For this review, take the finished solid that the model builds, in its own axes (mm). A direction names the side the tool comes from. Round coordinates to 2 decimals unless told otherwise and drop trailing zeros. Write each loop counter-clockwise with the first axis right and the second up, starting at its lowest first coordinate (ties: lowest second). Pieces come first, ordered by that corner, then holes. Notation, with made-up numbers: (65.5, -15.75) -> (119.5, -15.75) arc R26 ccw to (119.5, 1.25) -> close; hole circle Ø8 at (-28, 86). An arc over 180 degrees is marked (long way). Answer in a Markdown table with one row per item. Add a question column.
```python
from build123d import *
from OCP.BRepFilletAPI import BRepFilletAPI_MakeChamfer
from build123d.topology import SkipClean

# Parameters (mm, degrees)
SKETCH1_R                 = 12
SKETCH1_R_2               = 8
BOSS_EXTRUDE4_DEPTH       = 2
BOSS_EXTRUDE5_START       = 2
SKETCH1_9_R               = 12
SKETCH1_9_R_2             = 9
BOSS_EXTRUDE5_DEPTH       = 4
BOSS_EXTRUDE6_START       = 2
BOSS_EXTRUDE6_DEPTH       = 2
BOSS_EXTRUDE7_START       = 4
BOSS_EXTRUDE7_DEPTH       = 2
BOSS_EXTRUDE8_START       = 4
SKETCH1_12_W              = 60
SKETCH1_12_H              = 60
SKETCH1_12_R              = 12
BOSS_EXTRUDE8_DEPTH       = 2
BOSS_EXTRUDE9_DEPTH       = 6
CHAMFER1_SIZE             = 1
CHAMFER1_SIZE2            = 0.176326981
BOSS_EXTRUDE10_DEPTH      = 6
BOSS_EXTRUDE11_DEPTH      = 20
BOSS_EXTRUDE12_DEPTH      = 2
BOSS_EXTRUDE12_DEPTH_BACK = 2
SKETCH1_14_R              = 8
CUT_EXTRUDE1_DEPTH        = 46.343136195


with BuildPart() as part:
    # Sketch1 → Boss-Extrude4 (new body)
    with BuildSketch(Plane(origin=(0, 0, 0), x_dir=(1, 0, 0), z_dir=(0, 1, 0))):
        with Locations(Location((0, 0, 0), (0, 0, 270))):
            Circle(SKETCH1_R)
        with Locations(Location((0, 0, 0), (0, 0, 270))):
            Circle(SKETCH1_R_2, mode=Mode.SUBTRACT)
    extrude(amount=BOSS_EXTRUDE4_DEPTH)

    # Sketch1<9> → Boss-Extrude5 (add)
    with BuildSketch(Plane(origin=(0, 0, 0), x_dir=(1, 0, 0), z_dir=(0, 1, 0)).offset(BOSS_EXTRUDE5_START)):
        with Locations(Location((0, 0, 0), (0, 0, 270))):
            Circle(SKETCH1_9_R)
        with Locations(Location((0, 0, 0), (0, 0, 270))):
            Circle(SKETCH1_9_R_2, mode=Mode.SUBTRACT)
    extrude(amount=BOSS_EXTRUDE5_DEPTH)

    # Sketch1<10> → Boss-Extrude6 (add)
    with SkipClean():  # the faces are left unmerged after this step: merging them gives an invalid solid
        with BuildSketch(Plane(origin=(0, 0, 0), x_dir=(1, 0, 0), z_dir=(0, 1, 0)).offset(BOSS_EXTRUDE6_START)):
            with BuildLine():
                ThreePointArc((0, 8), (2.070552361, 7.72740661), (4, 6.92820323))
                Line((4, 6.92820323), (4.5, 7.794228634))
                ThreePointArc((4.5, 7.794228634), (2.329371406, 8.693332437), (0, 9))
                Line((0, 9), (0, 8))
            make_face()
            with BuildLine():
                ThreePointArc((-8, 0), (-7.72740661, 2.070552361), (-6.92820323, 4))
                Line((-6.92820323, 4), (-7.794228634, 4.5))
                ThreePointArc((-7.794228634, 4.5), (-8.693332437, 2.329371406), (-9, 0))
                Line((-9, 0), (-8, 0))
            make_face()
            with BuildLine():
                Line((0, -9), (0, -8))
                ThreePointArc((0, -8), (-2.070552361, -7.72740661), (-4, -6.92820323))
                Line((-4, -6.92820323), (-4.5, -7.794228634))
                ThreePointArc((-4.5, -7.794228634), (-2.329371406, -8.693332437), (0, -9))
            make_face()
            with BuildLine():
                Line((9, 0), (8, 0))
                ThreePointArc((8, 0), (7.72740661, -2.070552361), (6.92820323, -4))
                Line((6.92820323, -4), (7.794228634, -4.5))
                ThreePointArc((7.794228634, -4.5), (8.693332437, -2.329371406), (9, 0))
            make_face()
        extrude(amount=BOSS_EXTRUDE6_DEPTH)

    # Sketch1<11> → Boss-Extrude7 (add)
    with SkipClean():  # the faces are left unmerged after this step: merging them gives an invalid solid
        with BuildSketch(Plane(origin=(0, 0, 0), x_dir=(1, 0, 0), z_dir=(0, 1, 0)).offset(BOSS_EXTRUDE7_START)):
            with BuildLine():
                ThreePointArc((0, 8), (2.070552361, 7.72740661), (4, 6.92820323))
                Line((4, 6.92820323), (4.5, 7.794228634))
                ThreePointArc((4.5, 7.794228634), (2.329371406, 8.693332437), (0, 9))
                Line((0, 9), (0, 8))
            make_face()
            with BuildLine():
                ThreePointArc((4, 6.92820323), (5.656854249, 5.656854249), (6.92820323, 4))
                Line((6.92820323, 4), (7.794228634, 4.5))
                ThreePointArc((7.794228634, 4.5), (6.363961031, 6.363961031), (4.5, 7.794228634))
                Line((4.5, 7.794228634), (4, 6.92820323))
            make_face()
            with BuildLine():
                ThreePointArc((-8, 0), (-7.72740661, 2.070552361), (-6.92820323, 4))
                Line((-6.92820323, 4), (-7.794228634, 4.5))
                ThreePointArc((-7.794228634, 4.5), (-8.693332437, 2.329371406), (-9, 0))
                Line((-9, 0), (-8, 0))
            make_face()
            with BuildLine():
                ThreePointArc((-6.92820323, 4), (-5.656854249, 5.656854249), (-4, 6.92820323))
                Line((-4, 6.92820323), (-4.5, 7.794228634))
                ThreePointArc((-4.5, 7.794228634), (-6.363961031, 6.363961031), (-7.794228634, 4.5))
                Line((-7.794228634, 4.5), (-6.92820323, 4))
            make_face()
            with BuildLine():
                Line((-4.5, -7.794228634), (-4, -6.92820323))
                ThreePointArc((-4, -6.92820323), (-5.656854249, -5.656854249), (-6.92820323, -4))
                Line((-6.92820323, -4), (-7.794228634, -4.5))
                ThreePointArc((-7.794228634, -4.5), (-6.363961031, -6.363961031), (-4.5, -7.794228634))
            make_face()
            with BuildLine():
                Line((0, -9), (0, -8))
                ThreePointArc((0, -8), (-2.070552361, -7.72740661), (-4, -6.92820323))
                Line((-4, -6.92820323), (-4.5, -7.794228634))
                ThreePointArc((-4.5, -7.794228634), (-2.329371406, -8.693332437), (0, -9))
            make_face()
            with BuildLine():
                Line((9, 0), (8, 0))
                ThreePointArc((8, 0), (7.72740661, -2.070552361), (6.92820323, -4))
                Line((6.92820323, -4), (7.794228634, -4.5))
                ThreePointArc((7.794228634, -4.5), (8.693332437, -2.329371406), (9, 0))
            make_face()
            with BuildLine():
                Line((7.794228634, -4.5), (6.92820323, -4))
                ThreePointArc((6.92820323, -4), (5.656854249, -5.656854249), (4, -6.92820323))
                Line((4, -6.92820323), (4.5, -7.794228634))
                ThreePointArc((4.5, -7.794228634), (6.363961031, -6.363961031), (7.794228634, -4.5))
            make_face()
        extrude(amount=BOSS_EXTRUDE7_DEPTH)

    # Sketch1<12> → Boss-Extrude8 (add)
    with SkipClean():  # the faces are left unmerged after this step: merging them gives an invalid solid
        with BuildSketch(Plane(origin=(0, 0, 0), x_dir=(1, 0, 0), z_dir=(0, 1, 0)).offset(BOSS_EXTRUDE8_START)):
            Rectangle(SKETCH1_12_W, SKETCH1_12_H)
            with Locations(Location((0, 0, 0), (0, 0, 270))):
                Circle(SKETCH1_12_R, mode=Mode.SUBTRACT)
        extrude(amount=BOSS_EXTRUDE8_DEPTH)

    # Sketch3 → Boss-Extrude9 (add)
    with SkipClean():  # the faces are left unmerged after this step: merging them gives an invalid solid
        with BuildSketch(Plane.XZ.offset(-4)):
            Polygon((-30, -30), (30, -30), (30, -28), (-28, -28), (-28, 30), (-30, 30), align=None)
            Polygon((30, -20), (30, -18), (-18, -18), (-18, 30), (-20, 30), (-20, -20), align=None)
        extrude(amount=BOSS_EXTRUDE9_DEPTH)

    # Chamfer1: one chamfer whose edges measure the first distance from different faces: ONE call of the kernel's chamfer builder (chamfer() names one face for all edges)
    chamfer1_edges_1 = [part.edges().sort_by_distance(p)[0] for p in [
        (-28, -2, 1),
    ]]
    chamfer1_side_1 = [part.faces().sort_by_distance(p)[0] for p in [
        (-28, 1, 1),
    ]]
    chamfer1_edges_2 = [part.edges().sort_by_distance(p)[0] for p in [
        (1, -2, -28),
    ]]
    chamfer1_side_2 = [part.faces().sort_by_distance(p)[0] for p in [
        (1, 1, -28),
    ]]
    chamfer1_edges_3 = [part.edges().sort_by_distance(p)[0] for p in [
        (-29, -2, 30),
    ]]
    chamfer1_side_3 = [part.faces().sort_by_distance(p)[0] for p in [
        (-29, 1, 30),
    ]]
    chamfer1_edges_4 = [part.edges().sort_by_distance(p)[0] for p in [
        (-30, -2, 0),
    ]]
    chamfer1_side_4 = [part.faces().sort_by_distance(p)[0] for p in [
        (-30, 1, 0),
    ]]
    chamfer1_edges_5 = [part.edges().sort_by_distance(p)[0] for p in [
        (0, -2, -30),
    ]]
    chamfer1_side_5 = [part.faces().sort_by_distance(p)[0] for p in [
        (0, 1, -30),
    ]]
    chamfer1_edges_6 = [part.edges().sort_by_distance(p)[0] for p in [
        (30, -2, -29),
    ]]
    chamfer1_side_6 = [part.faces().sort_by_distance(p)[0] for p in [
        (30, 1, -29),
    ]]
    chamfer1 = BRepFilletAPI_MakeChamfer(part.part.solid().wrapped)
    for e in chamfer1_edges_1:
        chamfer1.Add(CHAMFER1_SIZE, CHAMFER1_SIZE2, e.wrapped, chamfer1_side_1[0].wrapped)  # the first distance lies on this face
    for e in chamfer1_edges_2:
        chamfer1.Add(CHAMFER1_SIZE, CHAMFER1_SIZE2, e.wrapped, chamfer1_side_2[0].wrapped)  # the first distance lies on this face
    for e in chamfer1_edges_3:
        chamfer1.Add(CHAMFER1_SIZE, CHAMFER1_SIZE2, e.wrapped, chamfer1_side_3[0].wrapped)  # the first distance lies on this face
    for e in chamfer1_edges_4:
        chamfer1.Add(CHAMFER1_SIZE, CHAMFER1_SIZE2, e.wrapped, chamfer1_side_4[0].wrapped)  # the first distance lies on this face
    for e in chamfer1_edges_5:
        chamfer1.Add(CHAMFER1_SIZE, CHAMFER1_SIZE2, e.wrapped, chamfer1_side_5[0].wrapped)  # the first distance lies on this face
    for e in chamfer1_edges_6:
        chamfer1.Add(CHAMFER1_SIZE, CHAMFER1_SIZE2, e.wrapped, chamfer1_side_6[0].wrapped)  # the first distance lies on this face
    add(Compound.cast(chamfer1.Shape()), mode=Mode.REPLACE)

    # Sketch6 → Boss-Extrude10 (add)
    with BuildSketch(Plane.XZ.offset(-4)):
        Polygon((-18, 30), (-18, 28), (28, 28), (28, -18), (30, -18), (30, 30), align=None)
    extrude(amount=BOSS_EXTRUDE10_DEPTH)

    # Sketch3<3> → Boss-Extrude11 (add)
    with BuildSketch(Plane.XZ.offset(-4)):
        Polygon((-20, 30), (-20, -20), (-18, -18), (-18, 28), (-18, 30), align=None)
        Polygon((-20, -20), (30, -20), (30, -18), (28, -18), (-18, -18), align=None)
    extrude(amount=BOSS_EXTRUDE11_DEPTH)

    # Sketch9 → Boss-Extrude12 (add, two sides: drawn at the far end of the back side and taken through both)
    with BuildSketch(Plane(origin=(0, 0, 0), x_dir=(-0.7071067811865476, 0, -0.7071067811865475), z_dir=(0.7071067811865475, 0, -0.7071067811865476)).offset(-BOSS_EXTRUDE12_DEPTH_BACK)):
        Polygon((25.455844123, -16), (25.455844123, 0), (0, 0), align=None)
    extrude(amount=BOSS_EXTRUDE12_DEPTH + BOSS_EXTRUDE12_DEPTH_BACK)

    # Sketch1<14> → Cut-Extrude1 (cut, through all)
    with SkipClean():  # the faces are left unmerged after this step: merging them gives an invalid solid
        with BuildSketch(Plane(origin=(0, 0, 0), x_dir=(1, 0, 0), z_dir=(0, 1, 0))):
            with Locations(Location((0, 0, 0), (0, 0, 90))):
                Circle(SKETCH1_14_R)
        extrude(amount=-CUT_EXTRUDE1_DEPTH, mode=Mode.SUBTRACT)
    add(part.part.scale(1), mode=Mode.REPLACE)  # the faces are merged on a copy


solid = part.part
```
1. We need section C-C (z = 2). Write out the cut boundary in (x, y).
2. We need section B-B (x = 2). Write out the cut boundary in (y, z), plus the area to 3 significant figures.
3. Tool access review of faces 1 (the flat face through (-6, 4, -6)), 2 (the flat face through (1, 2, -28)), 3 (the flat face through (28, 1, 5)), 4 (the flat face through (-11.671, -10.356, -11.631)): name each direction out of +Z, -Z, +X, -X, +Y, -Y from which nothing blocks a thin tool from reaching the whole face with its end or side.
4. The part is to be moulded in two halves that separate along Y. For faces 5 (the flat face through (17, -2, 29)), 6 (the flat face through (-10.77, -5.63, -13.6)), 7 (the cylindrical face through (-8.29, 3.53, 3.5)), say which applies: pulls with the +Y half, pulls with the -Y half, needs draft (parallel to the pull), parting line crosses it, or undercut.
5. For L1, parallel to Z at x = 19.5, y = 2.5; L2, parallel to X at y = -1.25, z = 0; L3, parallel to X at y = 1, z = 11, list the stretches that pass through material, from the lowest coordinate up. Write a range as [from, to].
6. Clearance check with flat-ended pins moving along their axes: pin 1 Ø1.1 at (x, z) = (-5, 6) entering from -Y; pin 2 Ø6 at (x, z) = (11, 20) entering from -Y; pin 3 Ø8 at (x, y) = (19.5, -7) entering from +Z. State where each tip first meets the part, or that it passes through.
7. We need section A-A (z = -24). Write out the cut boundary in (x, y).
8. We need section D-D (y = -6.25). Write out the cut boundary in (x, z), plus the area to 3 significant figures.
Response:
| question | item | result |
|---|---|---|
| 1 | outline | (-30, -1) -> (-29.82, -2) -> (-28.18, -2) -> (-28, -1) -> (-28, 4) -> (-20, 4) -> (-20, -16) -> (-18, -16) -> (-18, 4) -> (-11.83, 4) -> (-11.83, 0) -> (-7.75, 0) -> (-7.75, 2) -> (-8.77, 2) -> (-8.77, 6) -> (-30, 6) -> close; (7.75, 0) -> (11.83, 0) -> (11.83, 4) -> (28, 4) -> (28, -2) -> (30, -2) -> (30, 6) -> (7.75, 6) -> close |
| 2 | outline | (-16, -20) -> (4, -20) -> (4, -28) -> (-1, -28) -> (-2, -28.18) -> (-2, -29.82) -> (-1, -30) -> (6, -30) -> (6, -7.75) -> (0, -7.75) -> (0, -11.83) -> (4, -11.83) -> (4, -18) -> (-16, -18) -> close; (-2, 28) -> (4, 28) -> (4, 11.83) -> (0, 11.83) -> (0, 7.75) -> (2, 7.75) -> (2, 8.77) -> (6, 8.77) -> (6, 30) -> (-2, 30) -> close |
| 2 | area | 181 mm2 |
| 3 | face 1 | none |
| 3 | face 2 | +X, -Y |
| 3 | face 3 | -Y |
| 3 | face 4 | +Z, +X, -Y |
| 4 | face 5 | pulls with the -Y half |
| 4 | face 6 | needs draft |
| 4 | face 7 | undercut |
| 5 | L1 | [-30, -28], [-20, -18], [28, 30] |
| 5 | L2 | [-29.96, -28.04], [-20, -18], [28, 30] |
| 5 | L3 | [-30, -28], [-20, -18], [-4.8, 4.8], [28, 30] |
| 6 | pin 1 | y = 0 |
| 6 | pin 2 | y = 4 |
| 6 | pin 3 | z = -18 |
| 7 | outline | (-30, -1) -> (-29.82, -2) -> (-28.18, -2) -> (-28, -1) -> (-28, 4) -> (30, 4) -> (30, 6) -> (-30, 6) -> close |
| 8 | outline | (-20, -20) -> (30, -20) -> (30, -18) -> (-15.17, -18) -> (-5.62, -8.45) -> (-8.45, -5.62) -> (-18, -15.17) -> (-18, 30) -> (-20, 30) -> close |
| 8 | area | 254 mm2 |
